from build123d import *

# Parameters (mm, degrees)
CROQUIS3_R              = 25
SALIENTE_EXTRUIR2_DEPTH = 100
CROQUIS3_3_W            = 50
CROQUIS3_3_H            = 100
SALIENTE_EXTRUIR3_DEPTH = 30
CROQUIS4_R              = 7.5
CORTAR_EXTRUIR1_DEPTH   = 101


with BuildPart() as part:
    # Croquis3 → Saliente-Extruir2 (new body)
    with BuildSketch(Plane(origin=(0, 0, 0), x_dir=(1, 0, 0), z_dir=(0, 1, 0))):
        with BuildLine():
            Line((0, -50), (-50, -50))
            Line((-50, -50), (-50, -150))
            Line((-50, -150), (-100, -150))
            Line((-100, -150), (-100, 50))
            Line((-100, 50), (0, 50))
            ThreePointArc((0, 50), (50, 0), (0, -50))
        make_face()
        Circle(CROQUIS3_R, mode=Mode.SUBTRACT)
    extrude(amount=SALIENTE_EXTRUIR2_DEPTH)

    # Croquis3_3 → Saliente-Extruir3 (add)
    with BuildSketch(Plane(origin=(0, 0, 0), x_dir=(1, 0, 0), z_dir=(0, 1, 0))):
        with Locations((-25, -100)):
            Rectangle(CROQUIS3_3_W, CROQUIS3_3_H)
    extrude(amount=SALIENTE_EXTRUIR3_DEPTH)

    # Croquis4 → Cortar-Extruir1 (cut, through all)
    with BuildSketch(Plane(origin=(0, 0, 0), x_dir=(0, 0, -1), z_dir=(1, 0, 0))):
        with Locations((-130, 15)):
            Circle(CROQUIS4_R)
        with Locations((-70, 15)):
            Circle(CROQUIS4_R)
    extrude(amount=-CORTAR_EXTRUIR1_DEPTH, mode=Mode.SUBTRACT)


solid = part.part
Geometry: final body of the model. Coordinates: model frame, mm. A direction names the side the tool comes from. Coordinates: 2 decimals unless noted, no trailing zeros. Write each loop counter-clockwise with the first axis right and the second up, starting at its lowest first coordinate (ties: lowest second). Pieces come first, ordered by that corner, then holes. Notation, with made-up numbers: (38.5, -36) - (79.5, -36) arc R26 ccw to (79.5, 0) - close; hole circle Ø5 at (-12, 52.25). An arc over 180 degrees is marked (long way). Return JSON: item names as keys, results as strings.
Item 1: Section query A-A (y = 15). Output: boundary loops of the cut face in (x, z), and give its area (3 significant figures).
Completed:
{"outline": "(-100, -50) - (0, -50) arc R50 ccw to (0, 50) - (0, 62.5) - (-100, 62.5) - close; (-100, 77.5) - (0, 77.5) - (0, 122.5) - (-100, 122.5) - close; (-100, 137.5) - (0, 137.5) - (0, 150) - (-100, 150) - close; hole circle Ø50 at (0, 0)", "area": "19,000 mm2"}
Item 2: Pull-direction query (Z, two-part tool) for faces 4 (the face through (-62, 38, 150)), 5 (the face through (-49.3, 15.33, 77.493)), 6 (the face through (-41, 100, 26)); classes: +Z half, -Z half, draft (parallel to the pull), parting line (faces both ways), or undercut.
Completed:
{"face 4": "+Z half", "face 5": "undercut", "face 6": "draft"}
Item 3: Line query: L1, parallel to Z at x = -60, y = 8.5; L2, parallel to X at y = 66, z = 0; L3, parallel to Y at x = -28, z = 130. Output: solid intervals per line, ascending.
Completed:
{"L1": "z = -50 to 66.26, 73.74 to 126.26, 133.74 to 150", "L2": "x = -100 to -25, 25 to 50", "L3": "y = 0 to 7.5, 22.5 to 30"}
Item 4: Section query C-C (z = 70). Output: boundary loops of the cut face in (x, y).
Completed:
{"outline": "(-100, 0) - (0, 0) - (0, 7.5) - (-100, 7.5) - close; (-100, 22.5) - (0, 22.5) - (0, 30) - (-50, 30) - (-50, 100) - (-100, 100) - close"}
Item 5: Section query D-D (y = 93.5). Output: boundary loops of the cut face in (x, z).
Completed:
{"outline": "(-100, -50) - (0, -50) arc R50 ccw to (0, 50) - (-50, 50) - (-50, 150) - (-100, 150) - close; hole circle Ø50 at (0, 0)"}
Item 6: Pin query (flat end, axial travel): pin 1 Ø15 at (y, z) = (15, 92.5) entering from +X; pin 2 Ø1.5 at (y, z) = (50.5, 91) entering from +X; pin 3 Ø1 at (x, y) = (10, 79.5) entering from -Z. Return the tip coordinate at first contact, or that it passes through.
Completed:
{"pin 1": "stops at x = 0", "pin 2": "stops at x = -50", "pin 3": "stops at z = -49.09"}
Item 7: Reachability of faces 1 (the face through (0, 15, 101)), 2 (the face through (-100, 49, 51)), 3 (the face through (-25, 65, 50)) from +Z, -Z, +X, -X, +Y, -Y: full face, straight path, thin tool, end or side. Return the list, or none.
Completed:
{"face 1": "+Z, +X, +Y, -Y", "face 2": "+Z, -Z, -X, +Y, -Y", "face 3": "+Z, +X, +Y"}
Item 8: Section query B-B (x = -32.5). Output: boundary loops of the cut face in (y, z), and give its area (3 significant figures).
Completed:
{"outline": "(0, -50) - (100, -50) - (100, 50) - (30, 50) - (30, 150) - (0, 150) - close; hole circle Ø15 at (15, 70); hole circle Ø15 at (15, 130)", "area": "12,600 mm2"}
